Source: CAD feature listing. Evaluate the final solid. Frame: model axes, mm. Coordinates: 2 decimals unless noted, no trailing zeros. Order: outer loops, then holes, each group sorted by start corner. A loop starts at its lowest first (then second) coordinate and runs counter-clockwise, first axis right, second up.
```python
from build123d import *

# Parameters (mm, degrees)
SKETCH1_R           = 37.5
SKETCH1_R_2         = 2.5
SKETCH1_R_3         = 54.5
BOSS_EXTRUDE1_DEPTH = 3


with BuildPart() as part:
    # Sketch1 → Boss-Extrude1 (new body)
    with BuildSketch(Plane.XY):
        Circle(SKETCH1_R)
        Circle(SKETCH1_R_2, mode=Mode.SUBTRACT)
        with BuildLine():
            Line((225.97173913, 54.350925607), (-2.77173913, 37.397425877))
            ThreePointArc((-2.77173913, 37.397425877), (25.517736798, 27.478993953), (37.5, 0))
            ThreePointArc((37.5, 0), (25.517736798, -27.478993953), (-2.77173913, -37.397425877))
            Line((-2.77173913, -37.397425877), (225.97173913, -54.350925607))
            ThreePointArc((225.97173913, -54.350925607), (175.5, 0), (225.97173913, 54.350925607))
        make_face()
        with Locations((230, 0)):
            Circle(SKETCH1_R_3)
        with Locations((230, 0)):
            Circle(SKETCH1_R_2, mode=Mode.SUBTRACT)
    extrude(amount=BOSS_EXTRUDE1_DEPTH)


solid = part.part
```
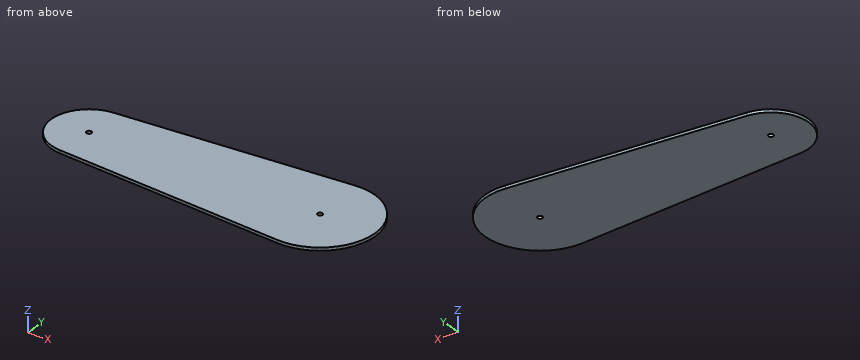
1. Ray query, line 1 (Y direction, x = 230, z = 0.6); line 2 (X direction, y = -1, z = 1.2); line 3 (Y direction, x = -3, z = 2.2). Return the intervals inside material, ascending.
Findings:
line 1: y = -54.5 to -2.5, 2.5 to 54.5
line 2: x = -37.49 to -2.29, 2.29 to 227.71, 232.29 to 284.49
line 3: y = -37.38 to 37.38
2. Section query A-A on z = 1.1. Return loops of the section in (x, y), plus the area to 3 significant figures.
Findings:
outline: (-2.77, -37.4) - (225.97, -54.35) arc R54.5 ccw (long way) to (225.97, 54.35) - (-2.77, 37.4) arc R37.5 ccw to start; hole circle Ø5 at (0, 0); hole circle Ø5 at (230, 0)
area: 28,100 mm2
3. Pin query (flat end, axial travel): P1, Ø1.5, axis at x = 123, z = 0.5, coming from the +Y side; P2, Ø1.5, axis at x = 186.5, y = 29.5, coming from the -Z side; P3, Ø4.5, axis at x = 230, y = 0, coming from the +Z side; P4, Ø1.5, axis at y = -2, z = 2.5, coming from the +X side. Return the tip coordinate at first contact, or that it passes through.
Findings:
P1: stops at y = 46.77
P2: stops at z = 0
P3: passes through
P4: stops at x = 284.49
4. Section query C-C on y = -43.5. Return loops of the section in (x, z).
Findings:
outline: (79.57, 0) - (262.83, 0) - (262.83, 3) - (79.57, 3) - close
5. Section query B-B on x = 212. Return loops of the section in (y, z), plus the area to 3 significant figures.
Findings:
outline: (-53.32, 0) - (53.32, 0) - (53.32, 3) - (-53.32, 3) - close
area: 320 mm2
